from build123d import *

# Parameters (mm, degrees)
SKETCH1_R               = 12.5
SKETCH1_R_2             = 4.5
BOSS_EXTRUDE1_DEPTH     = 1
SKETCH2_R               = 11
BOSS_EXTRUDE2_DEPTH     = 5
CUT_EXTRUDE1_DEPTH      = 19.371173071
CUT_EXTRUDE1_DEPTH_BACK = 19.371173071
SKETCH3_R               = 4.5


with BuildPart() as part:
    # Sketch1 → Boss-Extrude1 (new body)
    with BuildSketch(Plane(origin=(0, 0, 0), x_dir=(1, 0, 0), z_dir=(0, 1, 0))):
        with Locations(Location((0, 0, 0), (0, 0, 270))):
            Circle(SKETCH1_R)
        with Locations(Location((0, 0, 0), (0, 0, 270))):
            Circle(SKETCH1_R_2, mode=Mode.SUBTRACT)
    extrude(amount=BOSS_EXTRUDE1_DEPTH)

    # Sketch2 → Boss-Extrude2 (add)
    with BuildSketch(Plane(origin=(0, 1, 0), x_dir=(1, 0, 0), z_dir=(0, 1, 0))):
        with Locations(Location((0, 0, 0), (0, 0, 270))):
            Circle(SKETCH2_R)
    extrude(amount=BOSS_EXTRUDE2_DEPTH)

    # Sketch3 → Cut-Extrude1 (cut, two sides: drawn at the far end of the back side and taken through both)
    with BuildSketch(Plane.XZ.offset(-1).offset(-CUT_EXTRUDE1_DEPTH_BACK)):
        with Locations(Location((0, 0, 0), (0, 0, 270))):
            Circle(SKETCH3_R)
    extrude(amount=CUT_EXTRUDE1_DEPTH + CUT_EXTRUDE1_DEPTH_BACK, mode=Mode.SUBTRACT)


solid = part.part
Here's how the part is built. I have some questions about the finished solid (model axes, mm). A direction names the side the tool comes from. Round coordinates to 2 decimals unless told otherwise and drop trailing zeros. Write each loop counter-clockwise with the first axis right and the second up, starting at its lowest first coordinate (ties: lowest second). Pieces come first, ordered by that corner, then holes.
1. If we mould it in two halves opening along Z, with no side actions, what happens to faces 1 (the cylindrical face through (3.755, 0.493, 11.923)), 2 (the flat face through (-5, 0, 0)), 3 (the cylindrical face through (4.49, 3.04, -0.3))? For each: released by +Z, released by -Z, zero draft, split by the parting line, or undercut.
2. Suppose I cut it at C-C (x = 9). List the corners of the cut face in (y, z) for me.
3. I need wall thicknesses on L1, parallel to X at y = 2.5, z = 0; L2, parallel to Z at x = 1.5, y = 0.35; L3, parallel to Z at x = 1, y = 2.4. Which ranges of each line are inside material? Lowest first, please.
4. Suppose I cut it at A-A (x = 0). List the corners of the cut face in (y, z) for me.
5. Suppose I cut it at B-B (z = 0). List the corners of the cut face in (x, y) for me.
6. Will these pins go through, and if not, where does the flat tip stop? pin 1 Ø1 at (x, y) = (5.5, 4.5) entering from +Z; pin 2 Ø1.5 at (y, z) = (1.5, -2) entering from +X.
7. Suppose I cut it at D-D (y = 1.65). List the corners of the cut face in (x, z) for me.
8. For faces 4 (the flat face through (-10, 1, 5)), 5 (the flat face through (-5, 6, 0)), which set-ups out of +Z, -Z, +X, -X, +Y, -Y let a thin tool reach every point of the face, with its end or its side?
Answer sheet:
1. face 1: split by the parting line
1. face 2: zero draft
1. face 3: undercut
2. outline: (0, -8.67) - (1, -8.67) - (1, -6.32) - (6, -6.32) - (6, 6.32) - (1, 6.32) - (1, 8.67) - (0, 8.67) - close
3. L1: x = -11 to -4.5, 4.5 to 11
3. L2: z = -12.41 to -4.24, 4.24 to 12.41
3. L3: z = -10.95 to -4.39, 4.39 to 10.95
4. outline: (0, -12.5) - (1, -12.5) - (1, -11) - (6, -11) - (6, -4.5) - (0, -4.5) - close; (0, 4.5) - (6, 4.5) - (6, 11) - (1, 11) - (1, 12.5) - (0, 12.5) - close
5. outline: (-12.5, 0) - (-4.5, 0) - (-4.5, 6) - (-11, 6) - (-11, 1) - (-12.5, 1) - close; (4.5, 0) - (12.5, 0) - (12.5, 1) - (11, 1) - (11, 6) - (4.5, 6) - close
6. pin 1: stops at z = 9.8
6. pin 2: stops at x = 12.42
7. outline: circle Ø22 at (0, 0); hole circle Ø9 at (0, 0)
8. face 4: +Y
8. face 5: +Z, -Z, +X, -X, +Y
